Check sheet for the modelled part. Datum: model origin and axes. Units: mm. Face numbers are marked on the shaded views. A direction names the side the tool comes from. Round coordinates to 2 decimals unless told otherwise and drop trailing zeros. Order: outer loops, then holes, each group sorted by start corner. A loop starts at its lowest first (then second) coordinate and runs counter-clockwise, first axis right, second up. Notation, with made-up numbers: (24, 37) -> (44, 37) arc R20 ccw to (44, 65) -> close; hole circle Ø9 at (60, 35.5). An arc over 180 degrees is marked (long way). Answer in a Markdown table with one row per item.
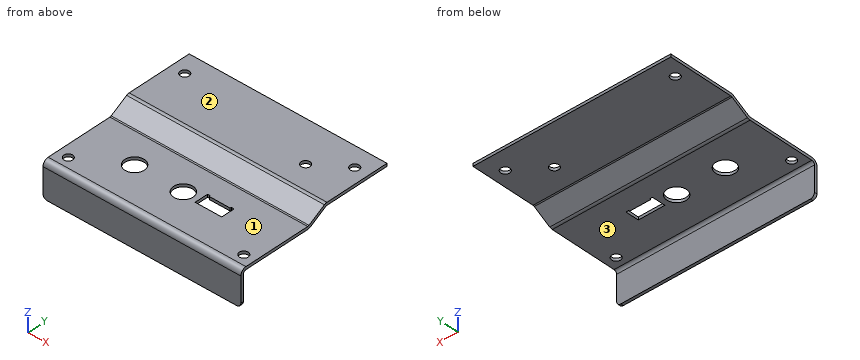
Autodesk Inventor part; units mm, degrees
ref_plane "YZ Plane" through (0, 0, 0) normal (1, 0, 0) x (0, 1, 0)
ref_plane "XZ Plane" through (0, 0, 0) normal (0, 1, 0) x (-1, 0, 0)
ref_plane "XY Plane" through (0, 0, 0) normal (0, 0, 1) x (1, 0, 0)
sketch "Sketch1" plane through (0, 0, 0) normal (0, 0, 1) x (1, 0, 0)
  line L0 (0, 18.2) -> (0, -18.2) construction
  line L1 (-49.7, 0) -> (49.7, 0) construction
  line L2 (-35.5, 13) -> (35.5, 13)
  line L3 (35.5, 13) -> (35.5, -13)
  line L4 (35.5, -13) -> (-35.5, -13)
  line L5 (-35.5, -13) -> (-35.5, 13)
  line L6 (-35.5, 13) -> (35.5, -13) construction
  line L7 (35.5, 13) -> (-35.5, -13) construction
  line L8 (14.985, 5.1105) -> (14.985, 5.5105)
  line L9 (14.985, 5.1105) -> (7.455, 5.1105)
  line L10 (7.455, 5.5105) -> (7.455, 5.1105)
  line L11 (6.455, 5.5105) -> (7.455, 5.5105)
  line L12 (6.455, 0.7105) -> (6.455, 5.5105)
  line L13 (6.455, 0.7105) -> (15.985, 0.7105)
  line L14 (15.985, 0.7105) -> (15.985, 5.5105)
  line L15 (14.985, 5.5105) -> (15.985, 5.5105)
  point P0 (0, 0)
  dimension "d0" = 71
  dimension "d1" = 26
extrude "Plate1" add sketch "Sketch1" along normal blind 1
sketch "Sketch2" plane through (-35.5, 13.5, 1.134) normal (0, 0.5, -0.8660254) x (-1, 0, 0)
  line L0 (-71, 0) -> (0, 0)
  line L1 (0, 0) -> (0, 7.4641)
  line L2 (0, 7.4641) -> (-71, 7.4641)
  line L3 (-71, 7.4641) -> (-71, 0)
edge flange "Flange1" height 8 angle 30 thickness 1 bend radius 1 thickness toward (0, 0.5, -0.8660254) relief tear relief width 1 relief depth 0.5 edges at (0, 13, 1) wall of the first edge with corners at (35.5, 13.5, 1.134) (-35.5, 13.5, 1.134) (-35.5, 19.9641, 4.866) (35.5, 19.9641, 4.866)
bend "Bend1"
corner "Corner1"
sketch "Sketch3" plane through (35.5, 19.9641, 3.866) normal (0, 0, 1) x (1, 0, 0)
  line L0 (-71, 0) -> (0, 0)
  line L1 (0, 0) -> (0, 23.869)
  line L2 (0, 23.869) -> (-71, 23.869)
  line L3 (-71, 23.869) -> (-71, 0)
edge flange "Flange2" height 23.869 angle 30 thickness 1 bend radius 1 thickness toward (0, 0, 1) relief tear relief width 1 relief depth 0.5 edges at (0, 20.4641, 4) wall of the first edge with corners at (-35.5, 19.9641, 3.866) (35.5, 19.9641, 3.866) (35.5, 43.8331, 3.866) (-35.5, 43.8331, 3.866)
bend "Bend2"
corner "Corner2"
sketch "Sketch4" plane through (-35.5, -12, 1) normal (0, -1, 0) x (1, 0, 0)
  line L0 (71, 0) -> (0, 0)
  line L1 (0, 0) -> (0, -12.5)
  line L2 (0, -12.5) -> (71, -12.5)
  line L3 (71, -12.5) -> (71, 0)
edge flange "Flange3" height 12.5 angle 90 thickness 1 bend radius 1 thickness toward (0, -1, 0) relief tear relief width 1 relief depth 0.5 edges at (0, -13, 0) wall of the first edge with corners at (35.5, -12, 1) (-35.5, -12, 1) (-35.5, -12, -11.5) (35.5, -12, -11.5)
bend "Bend3"
corner "Corner3"
fillet "Fillet1" radius 1.5 2 edges at (-35.5, -12.5, -11.5) (35.5, -12.5, -11.5)
sketch "Sketch5" plane through (-35.5, 43.8331, 4.866) normal (0, 0, 1) x (1, 0, 0)
  circle A0 centre (5, -7.1331) radius 1.6
  circle A1 centre (66, -7.1331) radius 1.6
  circle A2 centre (55.5, -14.8331) radius 1.5
  point P0 (35.5, -43.8331)
hole "Hole3" at (-30.5, 36.7, 4.866) at (20, 29, 4.866) at (30.5, 36.7, 4.866) direction (0, 0, -1) diameter 3.2 end through all
sketch "Sketch6" plane through (0, 0, 1) normal (0, 0, 1) x (1, 0, 0)
  circle A0 centre (-16.48, 2) radius 2.286
  circle A1 centre (1.02, 2) radius 2.286
  circle A2 centre (-31.5, -7.5) radius 1.6
  circle A3 centre (31.5, -7.5) radius 1.6
  point P0 (0, 0)
hole "Hole4" at (-31.5, -7.5, 1) at (31.5, -7.5, 1) direction (0, 0, -1) diameter 3.2 end through all
hole "Hole5" at (1.02, 2, 1) at (-16.48, 2, 1) direction (0, 0, -1) diameter 7 end through all
equation "\"d62\" = Thickness"
equation "\"d2\" = Thickness"
equation "\"d3\" = BendReliefWidth"
equation "\"d4\" = BendReliefDepth"
equation "\"d5\" = MinimumRemnant"
equation "\"d6\" = TransitionRadius"
equation "\"d9\" = BendRadius"
equation "\"d10\" = CornerReliefSize"
equation "\"d11\" = GapSize"
equation "\"d12\" = JacobiRadiusSize"
equation "\"d13\" = BendReliefWidth"
equation "\"d14\" = BendReliefDepth"
equation "\"d15\" = MinimumRemnant"
equation "\"d16\" = TransitionRadius"
equation "\"d19\" = BendRadius"
equation "\"d20\" = CornerReliefSize"
equation "\"d21\" = GapSize"
equation "\"d22\" = JacobiRadiusSize"
equation "\"d23\" = BendReliefWidth"
equation "\"d24\" = BendReliefDepth"
equation "\"d25\" = MinimumRemnant"
equation "\"d26\" = TransitionRadius"
equation "\"d29\" = BendRadius"
equation "\"d30\" = CornerReliefSize"
equation "\"d31\" = GapSize"
equation "\"d32\" = JacobiRadiusSize"
equation "\"BendRadius\" = Thickness"
equation "\"BendReliefWidth\" = Thickness"
equation "\"BendReliefDepth\" = 0.5 * Thickness"
equation "\"CornerReliefSize\" = 4 * Thickness"
equation "\"MinimumRemnant\" = 2 * Thickness"
equation "\"TransitionRadius\" = BendRadius"
equation "\"JacobiRadiusSize\" = BendRadius"
equation "\"GapSize\" = Thickness"
properties part number "Enclosure-Cap"
Item 1: Cross-section at D-D (z = -5). Record the boundary of the cut face in (x, y).
Result sheet:
| item | result |
|---|---|
| outline | (-35.5, -13) -> (35.5, -13) -> (35.5, -12) -> (-35.5, -12) -> close |
Item 2: Depth check by flat-ended pin: P1, Ø5, axis at y = 9.5, z = -0.5, coming from the +X side; P2, Ø12, axis at x = -15.5, y = 0.5, coming from the +Z side; P3, Ø0.5, axis at x = 15.5, z = 0.5, coming from the -Y side; P4, Ø12, axis at x = 6, y = 0.5, coming from the -Z side. Enter the tip coordinate at first touch or a pass-through.
Result sheet:
| item | result |
|---|---|
| P1 | stops at x = 35.5 |
| P2 | stops at z = 1 |
| P3 | stops at y = -12.56 |
| P4 | stops at z = 0 |
Item 3: Scan lines: line 1 (X direction, y = 36.7, z = 4.15); line 2 (X direction, y = 2, z = 0.85) (3 decimals); line 3 (Z direction, x = -17.5, y = -8.5). Record each from-to range of solid material in increasing order. Write a range as [from, to].
Result sheet:
| item | result |
|---|---|
| line 1 | x = [-35.5, -32.1], [-28.9, 28.9], [32.1, 35.5] |
| line 2 | x = [-35.5, -19.98], [-12.98, -2.48], [4.52, 6.455], [15.985, 35.5] |
| line 3 | z = [0, 1] |
Item 4: Cross-section at C-C (x = -16.48). Record the boundary of the cut face in (y, z).
Result sheet:
| item | result |
|---|---|
| outline | (-13, -11.5) -> (-12, -11.5) -> (-12, -1) arc R1 cw to (-11, 0) -> (-1.5, 0) -> (-1.5, 1) -> (-11, 1) arc R2 ccw to (-13, -1) -> close; (5.5, 0) -> (13, 0) arc R2 ccw to (14, 0.27) -> (20, 3.73) arc R1 cw to (20.5, 3.87) -> (43.83, 3.87) -> (43.83, 4.87) -> (20.5, 4.87) arc R2 ccw to (19.5, 4.6) -> (13.5, 1.13) arc R1 cw to (13, 1) -> (5.5, 1) -> close |
Item 5: Cross-section at A-A (y = 29). Record the boundary of the cut face in (x, z).
Result sheet:
| item | result |
|---|---|
| outline | (-35.5, 3.87) -> (18.4, 3.87) -> (18.4, 4.87) -> (-35.5, 4.87) -> close; (21.6, 3.87) -> (35.5, 3.87) -> (35.5, 4.87) -> (21.6, 4.87) -> close |
Item 6: Cross-section at B-B (y = 2). Record the boundary of the cut face in (x, z) (3 decimals).
Result sheet:
| item | result |
|---|---|
| outline | (-35.5, 0) -> (-19.98, 0) -> (-19.98, 1) -> (-35.5, 1) -> close; (-12.98, 0) -> (-2.48, 0) -> (-2.48, 1) -> (-12.98, 1) -> close; (4.52, 0) -> (6.455, 0) -> (6.455, 1) -> (4.52, 1) -> close; (15.985, 0) -> (35.5, 0) -> (35.5, 1) -> (15.985, 1) -> close |
Item 7: Set-up check for the marked faces 1, 2 and 3: record each of +Z, -Z, +X, -X, +Y, -Y from which the full face is reachable in a straight line by a thin tool's end or side.
Result sheet:
| item | result |
|---|---|
| face 1 | +Z, +X, -X, -Y |
| face 2 | +Z, +X, -X, +Y, -Y |
| face 3 | -Z, +X, -X, +Y |
